Check sheet for the modelled part. Datum: model origin and axes. Units: mm. A direction names the side the tool comes from. Give positions to 0.01 mm unless a question says otherwise; leave off trailing zeros. Order: outer loops, then holes, each group sorted by start corner. A loop starts at its lowest first (then second) coordinate and runs counter-clockwise, first axis right, second up.
from build123d import *

# Parameters (mm, degrees)
F0_W     = 38
F0_H     = 55
F1_DEPTH = 21
F3_DEPTH = 11
F4_R     = 5


with BuildPart() as f1:
    # F0 (on Top) → F1 (new body)
    with BuildSketch(Plane.XY):
        with Locations((11.086939, 2.041674)):
            Rectangle(F0_W, F0_H)
    extrude(amount=F1_DEPTH)

    # F2 (on face) → F3 (join)
    with BuildSketch(Plane(origin=(0, 29.541674, 0), x_dir=(-1, 0, 0), z_dir=(0, 1, 0))):
        with BuildLine():
            ThreePointArc((-11.086939, 0), (-3.662318, 3.075379), (-0.586939, 10.5))
            ThreePointArc((-0.586939, 10.5), (-3.662318, 17.924621), (-11.086939, 21))
            ThreePointArc((-11.086939, 21), (-21.586939, 10.5), (-11.086939, 0))
        make_face()
    extrude(amount=F3_DEPTH)

    # F4
    f4_edges = [f1.edges().sort_by_distance(p)[0] for p in [
        (-7.913061, 29.541674, 10.5),
        (30.086939, 29.541674, 10.5),
        (30.086939, -25.458326, 10.5),
        (-7.913061, -25.458326, 10.5),
    ]]
    fillet(f4_edges, radius=F4_R)


solid = f1.part
1) Material ranges on L1, parallel to Y at x = 5, z = 1.75; L2, parallel to Y at x = 28, z = 18.75; L3, parallel to X at y = 34.5, z = 4.5, recorded low to high.
Recorded:
L1: y = -25.46 to 29.54
L2: y = -24.52 to 28.61
L3: x = 2.47 to 19.7
2) Depth check by flat-ended pin: pin 1 Ø1.5 at (y, z) = (28, 4) entering from +X; pin 2 Ø8 at (x, y) = (4, 30.5) entering from +Z. Enter the tip coordinate at first touch or a pass-through.
Recorded:
pin 1: stops at x = 29.29
pin 2: stops at z = 21
3) Section check B-B, the plane x = 27. Record the cut outline in (y, z), then the cut area to 3 significant figures.
Recorded:
outline: (-25.08, 0) - (29.16, 0) - (29.16, 21) - (-25.08, 21) - close
area: 1,140 mm2
4) Section check C-C, the plane z = 12.25. Record the cut outline in (x, y), then the cut area to 3 significant figures.
Recorded:
outline: (-7.91, -20.46) arc R5 ccw to (-2.91, -25.46) - (25.09, -25.46) arc R5 ccw to (30.09, -20.46) - (30.09, 24.54) arc R5 ccw to (25.09, 29.54) - (21.44, 29.54) - (21.44, 40.54) - (0.73, 40.54) - (0.73, 29.54) - (-2.91, 29.54) arc R5 ccw to (-7.91, 24.54) - close
area: 2,300 mm2
5) Section check A-A, the plane z = 9. Record the cut outline in (x, y), then the cut area to 3 significant figures.
Recorded:
outline: (-7.91, -20.46) arc R5 ccw to (-2.91, -25.46) - (25.09, -25.46) arc R5 ccw to (30.09, -20.46) - (30.09, 24.54) arc R5 ccw to (25.09, 29.54) - (21.48, 29.54) - (21.48, 40.54) - (0.69, 40.54) - (0.69, 29.54) - (-2.91, 29.54) arc R5 ccw to (-7.91, 24.54) - close
area: 2,300 mm2
6) Set-up check for faces 1 (the face through (-1, 29.542, 10)), 2 (the face through (11, 2, 0)), 3 (the face through (23, 29.542, 10)): record each of +Z, -Z, +X, -X, +Y, -Y from which the full face is reachable in a straight line by a thin tool's end or side.
Recorded:
face 1: -X, +Y
face 2: -Z, +X, -X, +Y, -Y
face 3: +X, +Y
